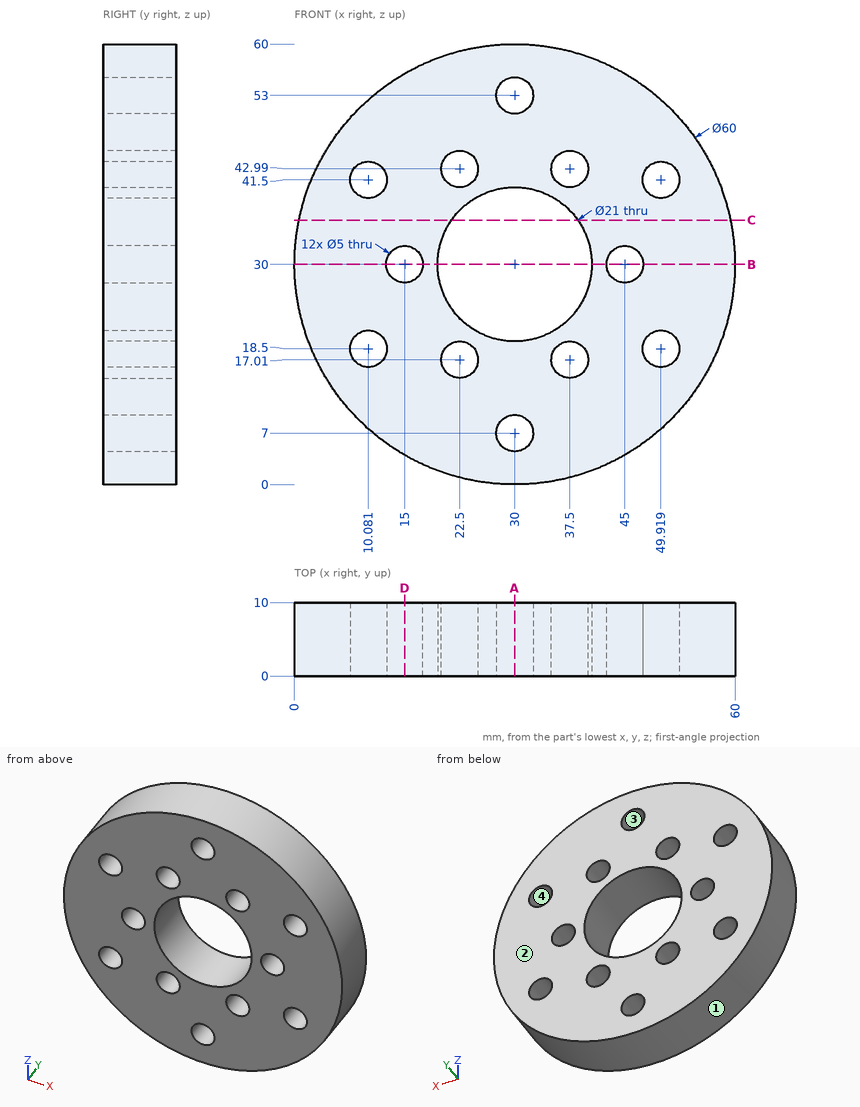
Print and shaded views of the part. All mm, measured from the part's lowest x, y and z. Give positions to 0.01 mm unless a question says otherwise; leave off trailing zeros. Order: outer loops, then holes, each group sorted by start corner. A loop starts at its lowest first (then second) coordinate and runs counter-clockwise, first axis right, second up. Notation, with made-up numbers: (10.5, -17.5) - (31.5, -17.5) arc R27 ccw to (31.5, 9.5) - close; hole circle Ø2 at (50.5, -34.5). An arc over 180 degrees is marked (long way). Use a Markdown table: item, result.
1) Saw through at C-C on z = 36. List the corners of the cut face in (x, y).
Checked values:
| item | result |
|---|---|
| outline | (0.61, 0) - (21.38, 0) - (21.38, 10) - (0.61, 10) - close; (38.62, 0) - (59.39, 0) - (59.39, 10) - (38.62, 10) - close |
2) Probe L1, parallel to Z at x = 38, y = 8 (1 decimal); L2, parallel to Z at x = 24, y = 0.5 (1 decimal); L3, parallel to Z at x = 49.5, y = 2 (1 decimal). List the from-to ranges inside material, lowest first. Write a range as from..to.
Checked values:
| item | result |
|---|---|
| L1 | 1.1..14.6, 19.5..23.2, 36.8..40.5, 45.4..58.9 |
| L2 | 0.6..15, 19..21.4, 38.6..41, 45..59.4 |
| L3 | 7.2..16, 21..39, 44..52.8 |
3) Saw through at D-D on x = 15. List the corners of the cut face in (y, z).
Checked values:
| item | result |
|---|---|
| outline | (0, 4.02) - (10, 4.02) - (10, 27.5) - (0, 27.5) - close; (0, 32.5) - (10, 32.5) - (10, 55.98) - (0, 55.98) - close |
4) Saw through at B-B on z = 30. List the corners of the cut face in (x, y).
Checked values:
| item | result |
|---|---|
| outline | (0, 0) - (12.5, 0) - (12.5, 10) - (0, 10) - close; (17.5, 0) - (19.5, 0) - (19.5, 10) - (17.5, 10) - close; (40.5, 0) - (42.5, 0) - (42.5, 10) - (40.5, 10) - close; (47.5, 0) - (60, 0) - (60, 10) - (47.5, 10) - close |
5) Two-plate mould, pull along Z, no slides. Class the marked faces 1, 2, 3 and 4: +Z half, -Z half, draft (parallel to the pull), parting line (faces both ways), or undercut.
Checked values:
| item | result |
|---|---|
| face 1 | parting line |
| face 2 | draft |
| face 3 | undercut |
| face 4 | undercut |
6) Flat gauge pins, fed straight in: P1, Ø4, axis at x = 50.5, y = 7.5, coming from the +Z side; P2, Ø3, axis at x = 49, y = 2.5, coming from the -Z side; P3, Ø1.5, axis at y = 2.5, z = 43, coming from the +X side (1 decimal). Where does each tip first touch, or does it go through?
Checked values:
| item | result |
|---|---|
| P1 | z = 53.62 |
| P2 | z = 5.63 |
| P3 | x = 57.4 |
7) Saw through at A-A on x = 30. List the corners of the cut face in (y, z).
Checked values:
| item | result |
|---|---|
| outline | (0, 0) - (10, 0) - (10, 4.5) - (0, 4.5) - close; (0, 9.5) - (10, 9.5) - (10, 19.5) - (0, 19.5) - close; (0, 40.5) - (10, 40.5) - (10, 50.5) - (0, 50.5) - close; (0, 55.5) - (10, 55.5) - (10, 60) - (0, 60) - close |
